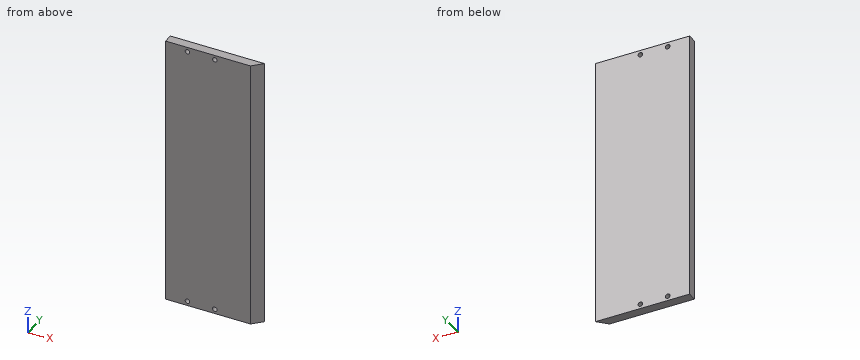
```python
from build123d import *

# Parameters (mm, degrees)
BOSS_EXTRUDE1_DEPTH   = 75
M3X0_5_TAPPED_HOLE1_D = 2.5


with BuildPart() as part:
    # Sketch1 → Boss-Extrude1 (new body, symmetric)
    with BuildSketch(Plane.XY):
        Polygon((51.57, 5), (46.53, 0), (0, 0), (0, 5), align=None)
    extrude(amount=BOSS_EXTRUDE1_DEPTH, both=True)

    # M3x0.5 Tapped Hole1 (through all)
    with Locations(Plane(origin=(0, 5, 0), x_dir=(1, 0, 0), z_dir=(0, 1, 0))):
        with Locations((12, -72.5), (27, -72.5)):
            m3x0_5_tapped_hole1 = Hole(M3X0_5_TAPPED_HOLE1_D / 2)

    # Mirror1: M3x0.5 Tapped Hole1 across plane
    add(m3x0_5_tapped_hole1.mirror(Plane.XY), mode=Mode.SUBTRACT)


solid = part.part
```
Here's how the part is built. I have some questions about the finished solid (model axes, mm). Coordinates: 2 decimals unless noted, no trailing zeros. Order: outer loops, then holes, each group sorted by start corner. A loop starts at its lowest first (then second) coordinate and runs counter-clockwise, first axis right, second up.
Item 1: If we section it at A-A, the plane y = 3.3: List the corners of the cut face in (x, z) for me, then the cut area to 3 significant figures.
Response values:
outline: (0, -75) - (49.86, -75) - (49.86, 75) - (0, 75) - close; hole circle Ø2.5 at (12, -72.5); hole circle Ø2.5 at (12, 72.5); hole circle Ø2.5 at (27, -72.5); hole circle Ø2.5 at (27, 72.5)
area: 7,460 mm2
Item 2: I need wall thicknesses on probe 1 along Z at (x, y) = (12, 2.4); probe 2 along Z at (x, y) = (11.5, 0.55); probe 3 along X at (y, z) = (1.9, -72.5). Which ranges of each line are inside material? Lowest first, please.
Response values:
probe 1: z = -75 to -73.75, -71.25 to 71.25, 73.75 to 75
probe 2: z = -75 to -73.65, -71.35 to 71.35, 73.65 to 75
probe 3: x = 0 to 10.75, 13.25 to 25.75, 28.25 to 48.45
Item 3: I'm going to push flat-ended pins straight in: pin 1 Ø4 at (x, z) = (12, -72.5) entering from +Y; pin 2 Ø1 at (y, z) = (3.5, -56) entering from +X; pin 3 Ø2 at (x, z) = (27, 72.5) entering from +Y; pin 4 Ø1.5 at (y, z) = (2, 51.5) entering from +X. Where does each tip first touch, or does it pass through?
Response values:
pin 1: stops at y = 5
pin 2: stops at x = 50.56
pin 3: passes through
pin 4: stops at x = 49.3
Item 4: If we section it at B-B, the plane z = -13.5: List the corners of the cut face in (x, y) for me.
Response values:
outline: (0, 0) - (46.53, 0) - (51.57, 5) - (0, 5) - close
